The model under review builds one solid part; all positions refer to its coordinate system, in mm. Face numbers are marked on the shaded views. A direction names the side the tool comes from. Coordinates: 2 decimals unless noted, no trailing zeros. Loops run counter-clockwise (first coordinate to the right, second up) from the corner with the lowest first, then second, coordinate; pieces in that order, holes last. Notation, with made-up numbers: (45, 79.25) - (49, 79.25) arc R22 ccw to (49, 108.25) - close; hole circle Ø7 at (-5, 32). An arc over 180 degrees is marked (long way). Answer in a Markdown table with one row per item. Add a question column.
(1) For P1, Ø3.5, axis at x = -0.5, z = -3, coming from the -Y side (3 decimals); P2, Ø2.5, axis at x = 0, z = -2.5, coming from the -Y side (3 decimals); P3, Ø2, axis at x = 1, y = -1.5, coming from the -Z side; P4, Ø5.5, axis at x = 0, y = -33.5, coming from the -Z side, all flat-tipped, find the tip position at first contact; note any pin that passes through.
(2) We need section A-A on z = -2.5. Write out the cut boundary in (x, y) (3 decimals).
(3) Machinability: for the marked faces 3, 4, 5 and 6, which of the approach directions +Z, -Z, +X, -X, +Y, -Y give a long, thin tool a straight path to every point of the face, cutting with its end or side? Answer none if there is none.
(4) We need section B-B on y = 0. Write out the cut boundary in (x, z), plus the area to 3 significant figures.
(5) For line 1 along Z through (x, y) = (0, -3.5); line 2 along Y through (x, z) = (-0.25, -5.5); line 3 along Z through (x, y) = (0, -9), list the stretches that pass through material, from the lowest coordinate up.
(6) We need section C-C on y = -18.5. Write out the cut boundary in (x, z).
(7) Mouldability with a two-part tool opening along Y and no side actions: class the marked faces 1 and 2 as +Y half, -Y half, draft (parallel to the pull), parting line (faces both ways), or undercut.
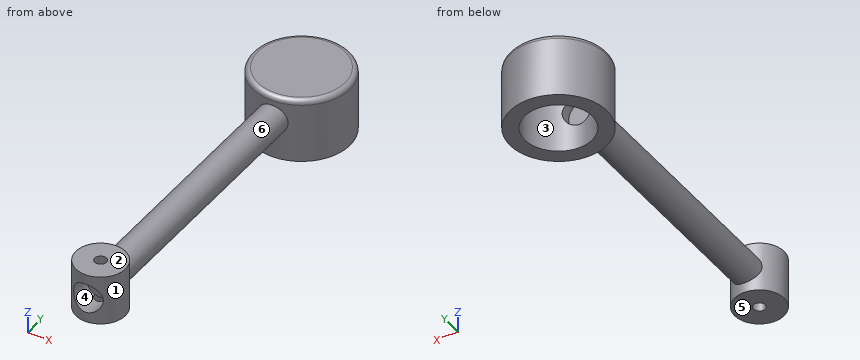
from build123d import *

# Parameters (mm, degrees)
SKETCH_1_R               = 4.9
EXTRUDE_1_DEPTH          = 6.5
SKETCH_7_R               = 3.4
CUT_EXTRUDE_1_DEPTH      = 5.5
SKETCH_8_R               = 1.5
CUT_EXTRUDE_6_DEPTH      = 5.9
FILLET_3_R               = 0.5
SKETCH_15_R              = 2.5
EXTRUDE_6_DEPTH          = 2.5
EXTRUDE_6_DEPTH_BACK     = 2.5
SKETCH_16_R              = 1.5
CUT_EXTRUDE_7_DEPTH      = 2.5
CUT_EXTRUDE_7_DEPTH_BACK = 2.5
SKETCH_17_R              = 0.6
CUT_EXTRUDE_8_DEPTH      = 7.5000001
SKETCH_18_R              = 1.5
EXTRUDE_7_DEPTH          = 29


with BuildPart() as part:
    # Sketch 1 → Extrude 1 (new body)
    with BuildSketch(Plane.XY):
        Circle(SKETCH_1_R)
    extrude(amount=-EXTRUDE_1_DEPTH)

    # Sketch 7 → Cut-Extrude 1 (cut)
    with BuildSketch(Plane(origin=(0, 0, -6.5), x_dir=(-1, 0, 0), z_dir=(0, 0, -1))):
        Circle(SKETCH_7_R)
    extrude(amount=-CUT_EXTRUDE_1_DEPTH, mode=Mode.SUBTRACT)

    # Sketch 8 → Cut-Extrude 6 (cut, through all)
    with BuildSketch(Plane(origin=(0, 0, 0), x_dir=(1, 0, 0), z_dir=(0, 1, 0))):
        with Locations(Location((0, 2.5, 0), (0, 0, 270))):  # turned: the seam where the file's is
            Circle(SKETCH_8_R)
    extrude(amount=-CUT_EXTRUDE_6_DEPTH, mode=Mode.SUBTRACT)

    # Fillet 3
    fillet_3_edges = [part.edges().sort_by_distance(p)[0] for p in [
        (-4.9, 0, 0),
    ]]
    fillet(fillet_3_edges, radius=FILLET_3_R)



with BuildPart() as body_2:
    # Sketch 15 → Extrude 6 (new body, two sides)
    with BuildSketch(Plane.XY.offset(-2.5)) as extrude_6_sk:
        with Locations((0, -33.125)):
            Circle(SKETCH_15_R)
    extrude(amount=EXTRUDE_6_DEPTH)
    extrude(extrude_6_sk.sketch, amount=-EXTRUDE_6_DEPTH_BACK)

    # Sketch 16 → Cut-Extrude 7 (cut, two sides)
    with BuildSketch(Plane(origin=(0, -33.125, 0), x_dir=(1, 0, 0), z_dir=(0, 1, 0))) as cut_extrude_7_sk:
        with Locations(Location((0, 2.5, 0), (0, 0, 270))):  # turned: the seam where the file's is
            Circle(SKETCH_16_R)
    extrude(amount=CUT_EXTRUDE_7_DEPTH, mode=Mode.SUBTRACT)
    extrude(cut_extrude_7_sk.sketch, amount=-CUT_EXTRUDE_7_DEPTH_BACK, mode=Mode.SUBTRACT)

    # Sketch 17 → Cut-Extrude 8 (cut, through all)
    with BuildSketch(Plane.XY):
        with Locations((0, -33.125)):
            Circle(SKETCH_17_R)
    extrude(amount=-CUT_EXTRUDE_8_DEPTH, mode=Mode.SUBTRACT)


with BuildPart() as part_1:
    add(part.part)

    add(body_2.part)  # Extrude 7 merges body 2
    # Sketch 18 → Extrude 7 (add)
    with BuildSketch(Plane(origin=(0, -33.125, 0), x_dir=(1, 0, 0), z_dir=(0, 1, 0))):
        with Locations(Location((0, 2.5, 0), (0, 0, 270))):  # turned: the seam where the file's is
            Circle(SKETCH_18_R)
    extrude(amount=EXTRUDE_7_DEPTH)


solid = part_1.part
Outcome:
| question | item | result |
|---|---|---|
| 1 | P1 | y = -35.625 |
| 1 | P2 | y = -33.125 |
| 1 | P3 | z = -1 |
| 1 | P4 | z = -5 |
| 2 | outline | (-1.5, -35.125) - (-1.5, -33.125) - (1.5, -33.125) - (1.5, -35.125) arc R2.5 ccw to (1.5, -31.125) - (1.5, -4.665) arc R4.9 ccw (long way) to (-1.5, -4.665) - (-1.5, -31.125) arc R2.5 ccw to start; hole (-1.5, -4.125) - (1.5, -4.125) - (1.5, -3.051) arc R3.4 ccw (long way) to (-1.5, -3.051) - close |
| 3 | face 3 | -Z |
| 3 | face 4 | -Y |
| 3 | face 5 | -Z, +X, -X, -Y |
| 3 | face 6 | none |
| 4 | outline | (-4.9, -6.5) - (-3.4, -6.5) - (-3.4, -1) - (3.4, -1) - (3.4, -6.5) - (4.9, -6.5) - (4.9, -0.5) arc R0.5 ccw to (4.4, 0) - (-4.4, 0) arc R0.5 ccw to (-4.9, -0.5) - close |
| 4 | area | 26.2 mm² |
| 5 | line 1 | -6.5 to -4, -1 to 0 |
| 5 | line 2 | -4.89 to -3.39, 3.39 to 4.89 |
| 5 | line 3 | -4 to -1 |
| 6 | outline | circle Ø3 at (0, -2.5) |
| 7 | face 1 | undercut |
| 7 | face 2 | draft |
